from build123d import *

# Parameters (mm, degrees)
CROQUIS1_R              = 13.5
CROQUIS1_R_2            = 10
SALIENTE_EXTRUIR1_DEPTH = 20
CHAFL_N1_SIZE           = 1
CHAFL_N2_SIZE           = 0.5


with BuildPart() as part:
    # Croquis1 → Saliente-Extruir1 (new body)
    with BuildSketch(Plane.XY):
        Circle(CROQUIS1_R)
        Circle(CROQUIS1_R_2, mode=Mode.SUBTRACT)
    extrude(amount=SALIENTE_EXTRUIR1_DEPTH)

    # Chaflán1
    chafl_n1_edges = [part.edges().sort_by_distance(p)[0] for p in [
        (-13.5, 0, 0),
        (-13.5, 0, 20),
    ]]
    chamfer(chafl_n1_edges, length=CHAFL_N1_SIZE)

    # Chaflán2
    chafl_n2_edges = [part.edges().sort_by_distance(p)[0] for p in [
        (-10, 0, 0),
        (-10, 0, 20),
    ]]
    chamfer(chafl_n2_edges, length=CHAFL_N2_SIZE)


solid = part.part
Input: part model. Units: mm. Frame: model coordinates. Coordinates: 2 decimals unless noted, no trailing zeros. Order: outer loops, then holes, each group sorted by start corner. A loop starts at its lowest first (then second) coordinate and runs counter-clockwise, first axis right, second up.
1. Cut plane C-C, the plane z = 13.5. Return loops of the section in (x, y).
Checked values:
outline: circle Ø27 at (0, 0); hole circle Ø20 at (0, 0)
2. Ray query, line 1 along Y through (x, z) = (0, 5.25); line 2 along X through (y, z) = (-9, 11); line 3 along X through (y, z) = (3, 1.5). Return the intervals inside material, ascending.
Checked values:
line 1: y = -13.5 to -10, 10 to 13.5
line 2: x = -10.06 to -4.36, 4.36 to 10.06
line 3: x = -13.16 to -9.54, 9.54 to 13.16
3. Cut plane A-A, the plane x = 0. Return loops of the section in (y, z), plus the area to 4 significant figures.
Checked values:
outline: (-13.5, 1) - (-12.5, 0) - (-10.5, 0) - (-10, 0.5) - (-10, 19.5) - (-10.5, 20) - (-12.5, 20) - (-13.5, 19) - close; (10, 0.5) - (10.5, 0) - (12.5, 0) - (13.5, 1) - (13.5, 19) - (12.5, 20) - (10.5, 20) - (10, 19.5) - close
area: 137.5 mm2
4. Contact query for flat-ended pins moving along their axis: P1, Ø1, axis at x = 5.5, z = 13.5, coming from the +Y side; P2, Ø2, axis at x = -2.5, z = 4, coming from the -Y side; P3, Ø8, axis at y = 8.5, z = 8.5, coming from the -X side; P4, Ø5, axis at x = 1, y = 10, coming from the -Z side. Output: stop coordinate, or through.
Checked values:
P1: stops at y = 12.54
P2: stops at y = -13.42
P3: stops at x = -12.73
P4: stops at z = 0
5. Draft query along X for faces 1 (the cylindrical face through (-2.93, -13.18, 9.87)), 2 (the cylindrical face through (-2.17, -9.76, 9.87)). Return one class per face: +X half, -X half, draft (parallel to the pull), parting line (faces both ways), or undercut.
Checked values:
face 1: parting line
face 2: undercut
